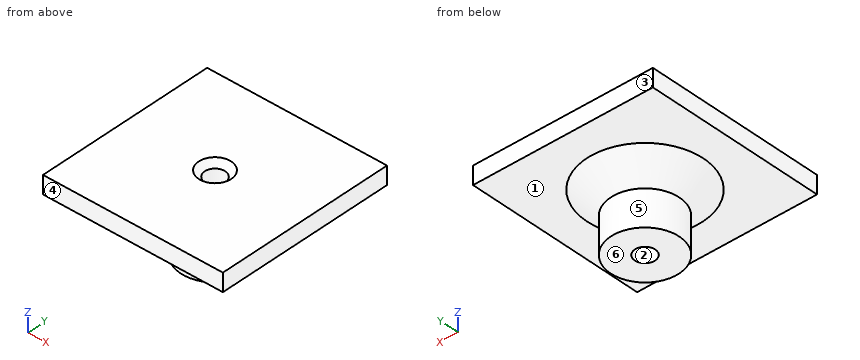
```python
from build123d import *

# Parameters (mm, degrees)
SKETCH_2_W          = 15
SKETCH_2_H          = 15
EXTRUDE_358_DEPTH   = 1.5
SKETCH_3_R          = 2.85
SKETCH_3_R_2        = 0.85
EXTRUDE_486_DEPTH   = 5
CHAMFER_1_SIZE      = 2
SKETCH_5_R          = 0.85
CUT_EXTRUDE_2_DEPTH = 12.7260394
CHAMFER_3_SIZE      = 0.5


with BuildPart() as part:
    # Эскиз2 → Extrude 358 (new body)
    with BuildSketch(Plane.XY):
        Rectangle(SKETCH_2_W, SKETCH_2_H)
    extrude(amount=EXTRUDE_358_DEPTH)

    # Эскиз3 → Extrude 486 (add)
    with BuildSketch(Plane.XY):
        Circle(SKETCH_3_R)
        Circle(SKETCH_3_R_2, mode=Mode.SUBTRACT)
    extrude(amount=-EXTRUDE_486_DEPTH)

    # Фаска1
    chamfer_1_edges = [part.edges().sort_by_distance(p)[0] for p in [
        (-2.85, 0, 0),
    ]]
    chamfer(chamfer_1_edges, length=CHAMFER_1_SIZE)

    # Эскиз5 → Вырез-Вытянуть2 (cut, through all)
    with BuildSketch(Plane.XY):
        Circle(SKETCH_5_R)
    extrude(amount=CUT_EXTRUDE_2_DEPTH, mode=Mode.SUBTRACT)

    # Фаска3
    chamfer_3_edges = [part.edges().sort_by_distance(p)[0] for p in [
        (-0.85, 0, 1.5),
    ]]
    chamfer(chamfer_3_edges, length=CHAMFER_3_SIZE)


solid = part.part
```
Geometry: final body of the model. Coordinates: model frame, mm. Face numbers are marked on the shaded views. A direction names the side the tool comes from. Round coordinates to 2 decimals unless told otherwise and drop trailing zeros. Loops run counter-clockwise (first coordinate to the right, second up) from the corner with the lowest first, then second, coordinate; pieces in that order, holes last. Notation, with made-up numbers: (9, 2.5) -> (47, 2.5) arc R25 ccw to (47, 25.5) -> close; hole circle Ø2 at (11, 55). An arc over 180 degrees is marked (long way). Use one line per item in the form item = value. Start each with the question number.
1) Section A-A on y = 0. Output: boundary loops of the cut face in (x, z).
2) Section D-D on y = -5.5. Output: boundary loops of the cut face in (x, z).
3) Access query for the marked faces 5 and 6. Directions: +Z, -Z, +X, -X, +Y, -Y. A direction counts if a zero-diameter tool reaches every point of the face in a straight line with its end or side. Return the directions, or none.
4) Draft query along Y for the marked faces 1, 2, 3 and 4. Return one class per face: released by +Y, released by -Y, zero draft, split by the parting line, or undercut.
5) Section C-C on z = -2.75. Output: boundary loops of the cut face in (x, y).
6) Line query: L1, parallel to Y at x = 0, z = -2.3; L2, parallel to Z at x = 5, y = -1.5; L3, parallel to X at y = 0, z = -1.9. Output: solid intervals per line, ascending.
7) First-contact query: P1, Ø3, axis at y = -0.5, z = -2.5, coming from the +X side; P2, Ø2, axis at y = -1, z = -2, coming from the -X side. Flat tips, straight axial feed; report the tip coordinate or a pass-through.
Response:
q1.outline = (-7.5, 0) -> (-4.85, 0) -> (-2.85, -2) -> (-2.85, -5) -> (-0.85, -5) -> (-0.85, 1) -> (-1.35, 1.5) -> (-7.5, 1.5) -> close; (0.85, -5) -> (2.85, -5) -> (2.85, -2) -> (4.85, 0) -> (7.5, 0) -> (7.5, 1.5) -> (1.35, 1.5) -> (0.85, 1) -> close
q2.outline = (-7.5, 0) -> (7.5, 0) -> (7.5, 1.5) -> (-7.5, 1.5) -> close
q3.face_5 = -Z
q3.face_6 = -Z, +X, -X, +Y, -Y
q4.face_1 = zero draft
q4.face_2 = undercut
q4.face_3 = released by +Y
q4.face_4 = released by -Y
q5.outline = circle Ø5.7 at (0, 0); hole circle Ø1.7 at (0, 0)
q6.L1 = -2.85 to -0.85, 0.85 to 2.85
q6.L2 = 0 to 1.5
q6.L3 = -2.95 to -0.85, 0.85 to 2.95
q7.P1 = 3.83
q7.P2 = -3.75
